Can you work these out from the model? Positions are in its coordinate system, mm. A direction names the side the tool comes from. Give positions to 0.01 mm unless a question says otherwise; leave off trailing zeros. Loops run counter-clockwise (first coordinate to the right, second up) from the corner with the lowest first, then second, coordinate; pieces in that order, holes last. Notation, with made-up numbers: (-0.5, -6.5) - (52.5, -6.5) arc R22 cw to (52.5, 31.5) - close; hole circle Ø9 at (43.5, 14). An arc over 180 degrees is marked (long way). Answer as a JSON object with one key per item and string values.
Autodesk Inventor part; units mm, degrees
ref_plane "YZ Plane" through (0, 0, 0) normal (1, 0, 0) x (0, 1, 0)
ref_plane "XZ Plane" through (0, 0, 0) normal (0, 1, 0) x (-1, 0, 0)
ref_plane "XY Plane" through (0, 0, 0) normal (0, 0, 1) x (1, 0, 0)
sketch "Sketch1" plane through (0, 0, 0) normal (0, 0, 1) x (1, 0, 0)
  circle A0 centre (0, 0) radius 2.5
  circle A1 centre (0, 0) radius 5
  line L0 (2.8292, -5) -> (-2.9155, -4.9502)
  line L1 (-2.9155, -4.9502) -> (-5.7447, 0.0498)
  line L2 (-5.7447, 0.0498) -> (-2.8292, 5)
  line L3 (-2.8292, 5) -> (2.9155, 4.9502)
  line L4 (2.9155, 4.9502) -> (5.7447, -0.0498)
  line L5 (5.7447, -0.0498) -> (2.8292, -5)
  dimension "d0" = 5
  dimension "d1" = 10
extrude "Extrusion1" add sketch "Sketch1" along normal blind 3 contours A0 | A1 L5 L0 L1 L2 L3 L4 | A1 L4 L5 | A1 L3 L4 | L5 L0 A1 | A1 L2 L3 | L0 L1 A1 | A1 L1 L2
sketch "Sketch2" plane through (0, 0, 3) normal (0, 0, 1) x (1, 0, 0)
  circle A0 centre (0, 0) radius 2.5
  dimension "d4" = 5
extrude "Extrusion2" add sketch "Sketch2" along normal blind 15
thread "Thread1"
sketch "Sketch3" plane through (0, 0, 0) normal (0, 0, -1) x (-1, 0, 0)
  point P0 (0, 0)
properties part number "Screw"
1) Imagine slicing it at A-A on x = 0. Write out the boundary of the cut face in (y, z), and give its area (3 significant figures).
Check sheet entries:
{"outline": "(-4.98, 0) - (4.98, 0) - (4.98, 3) - (2.5, 3) - (2.5, 18) - (-2.5, 18) - (-2.5, 3) - (-4.98, 3) - close", "area": "105 mm2"}
2) Imagine slicing it at B-B on z = 1.75. Write out the boundary of the cut face in (x, y).
Check sheet entries:
{"outline": "(-5.74, 0.05) - (-2.92, -4.95) - (2.83, -5) - (5.74, -0.05) - (2.92, 4.95) - (-2.83, 5) - close"}
3) Imagine slicing it at D-D on z = 12. Write out the boundary of the cut face in (x, y), and give its area (3 significant figures).
Check sheet entries:
{"outline": "circle Ø5 at (0, 0)", "area": "19.6 mm2"}
4) I need wall thicknesses on L1, parallel to Z at x = -3.5, y = 3; L2, parallel to X at y = -0.25, z = 8.75; L3, parallel to Y at x = -2, z = 14. Which ranges of each line are inside material? Lowest first, please.
Check sheet entries:
{"L1": "0 to 3", "L2": "-2.49 to 2.49", "L3": "-1.5 to 1.5"}
5) Imagine slicing it at C-C on y = 4.25. Write out the boundary of the cut face in (x, z).
Check sheet entries:
{"outline": "(-3.27, 0) - (3.31, 0) - (3.31, 3) - (-3.27, 3) - close"}
6) Which directions (+Z, -Z, +X, -X, +Y, -Y) give clear straight access to the entire face, cutting with the end or side of a thin tool? Please do faces 1 (the flat face through (4.3, 2.5, 1.5)), 2 (the cylindrical face through (-0.54, 2.44, 10.4)).
Check sheet entries:
{"face 1": "+Z, -Z, +X, +Y", "face 2": "+Z"}
7) I'm going to push flat-ended pins straight in: P1, Ø4, axis at x = 4, z = 14.5, coming from the -Y side; P2, Ø1, axis at y = 1, z = 4.5, coming from the -X side; P3, Ø3, axis at x = 1.5, z = 15, coming from the +Y side. Where does each tip first touch, or does it pass through?
Check sheet entries:
{"P1": "y = -1.5", "P2": "x = -2.45", "P3": "y = 2.5"}
